Read the model definition and answer for the solid it produces. Units are mm, in the model's axes. A direction names the side the tool comes from. Coordinates: 2 decimals unless noted, no trailing zeros. Loops run counter-clockwise (first coordinate to the right, second up) from the corner with the lowest first, then second, coordinate; pieces in that order, holes last. Notation, with made-up numbers: (29.5, 37.5) -> (68.5, 37.5) arc R21 ccw to (68.5, 44.5) -> close; hole circle Ø5 at (-28, 44.25). An arc over 180 degrees is marked (long way). Answer in a Markdown table with one row per item.
```python
from build123d import *

# Parameters (mm, degrees)
ESQUISSE1_W              = 330
ESQUISSE1_H              = 370
CORP_DEPTH               = 40
CONG_AVANT_RADIUS        = 165
CONG_AVANT_LENGTH        = 40
TROU_POUR_ROUE_DEPTH     = 38
ESQUISSE4_R              = 2
TROU_POUR_ROULETTE_DEPTH = 50
TROU_POUR_BALAYEUR_DEPTH = 25
MOTEUR_PALE_DEPTH        = 6.3
ESQUISSE7_R              = 3
ENL_V_MAT_EXTRU_10_DEPTH = 6.3
ESQUISSE8_W              = 6
ESQUISSE8_H              = 3.075554286
ENL_V_MAT_EXTRU_11_DEPTH = 6.3
ESQUISSE9_R              = 19.061984771
ENL_V_MAT_EXTRU_12_DEPTH = 33


with BuildPart() as part:
    # Esquisse1 → corp (new body)
    with BuildSketch(Plane(origin=(0, 0, 0), x_dir=(1, 0, 0), z_dir=(0, 1, 0))):
        with Locations((165, 185)):
            Rectangle(ESQUISSE1_W, ESQUISSE1_H)
    extrude(amount=CORP_DEPTH)

    # congé avant: full round fillet: the end face becomes a half cylinder, R = half its width
    cong_avant_face = Plane((165, 20, -370), x_dir=(0, 1, 0), z_dir=(0, 0, -1))  # on the end face: x along it, z out of the body
    cong_avant_slab = cong_avant_face.offset(-CONG_AVANT_RADIUS / 2) * Box(CONG_AVANT_LENGTH, 2 * CONG_AVANT_RADIUS, CONG_AVANT_RADIUS, mode=Mode.PRIVATE)  # the body's end, R deep
    cong_avant_round = Plane((165, 20, -205), x_dir=(0, 0, -1), z_dir=(0, 1, 0)) * Cylinder(CONG_AVANT_RADIUS, CONG_AVANT_LENGTH, mode=Mode.PRIVATE)  # its axis R under the face
    add(cong_avant_slab - cong_avant_round, mode=Mode.SUBTRACT)

    # Esquisse3 → trou pour roue (cut)
    with BuildSketch(Plane(origin=(0, 40, 0), x_dir=(1, 0, 0), z_dir=(0, 1, 0))):
        Polygon((46, 124), (46, 135), (0, 135), (0, 0), (46, 0), (46, 59.234399469), (54.724206143, 59.234399469), (54.724206143, 75), (46, 75), (46, 95), (61, 95), (61, 124), align=None)
        Polygon((284, 95), (284, 75), (275.275793857, 75), (275.275793857, 59.234399469), (284, 59.234399469), (284, 0), (330, 0), (330, 135), (284, 135), (284, 124), (269, 124), (269, 95), align=None)
    extrude(amount=-TROU_POUR_ROUE_DEPTH, mode=Mode.SUBTRACT)

    # Esquisse4 → trou pour roulette (cut)
    with BuildSketch(Plane(origin=(0, 40, 0), x_dir=(1, 0, 0), z_dir=(0, 1, 0))):
        with Locations(Location((176.95, 352.458632269, 0), (0, 0, 270))):
            Circle(ESQUISSE4_R)
        with Locations(Location((176.95, 323.158632269, 0), (0, 0, 90))):
            Circle(ESQUISSE4_R)
        with Locations(Location((153.05, 323.158632269, 0), (0, 0, 270))):
            Circle(ESQUISSE4_R)
        with Locations(Location((153.05, 352.458632269, 0), (0, 0, 90))):
            Circle(ESQUISSE4_R)
    extrude(amount=-TROU_POUR_ROULETTE_DEPTH, mode=Mode.SUBTRACT)

    # Esquisse5 → Trou pour balayeur (cut)
    with BuildSketch(Plane(origin=(0, 40, 0), x_dir=(1, 0, 0), z_dir=(0, 1, 0))):
        with BuildLine():
            Line((90, 286), (240, 286))
            ThreePointArc((240, 286), (309.290964938, 239.701257427), (293.033008589, 157.966991411))
            Line((293.033008589, 157.966991411), (240, 104.933982822))
            Line((240, 104.933982822), (240, 0))
            Line((240, 0), (90, 0))
            Line((90, 0), (90, 104.933982822))
            Line((90, 104.933982822), (36.966991411, 157.966991411))
            ThreePointArc((36.966991411, 157.966991411), (20.709035062, 239.701257427), (90, 286))
        make_face()
    extrude(amount=-TROU_POUR_BALAYEUR_DEPTH, mode=Mode.SUBTRACT)

    # Esquisse6 → moteur pale (cut)
    with BuildSketch(Plane(origin=(0, 15, 0), x_dir=(1, 0, 0), z_dir=(0, 1, 0))):
        with BuildLine():
            Line((257.506073255, 187.1), (255.885842754, 211))
            ThreePointArc((255.885842754, 211), (251.445088501, 222.191160152), (240.245274455, 226.610043405))
            ThreePointArc((240.245274455, 226.610043405), (240.122739998, 226.602511903), (240, 226.6))
            ThreePointArc((240, 226.6), (229.088615697, 221.822854824), (224.114157246, 211))
            Line((224.114157246, 211), (222.506073255, 187.1))
            ThreePointArc((222.506073255, 187.1), (227.152012558, 174.508282489), (239.63580106, 169.57967959))
            ThreePointArc((239.63580106, 169.57967959), (239.977179555, 169.600029468), (240.318655983, 169.581395004))
            ThreePointArc((240.318655983, 169.581395004), (252.842661862, 174.484702191), (257.506073255, 187.1))
        make_face()
        with BuildLine():
            ThreePointArc((89.754725545, 226.610043405), (78.554911499, 222.191160152), (74.114157246, 211))
            Line((74.114157246, 211), (72.493926745, 187.1))
            ThreePointArc((72.493926745, 187.1), (77.157338138, 174.484702191), (89.681344017, 169.581395004))
            ThreePointArc((89.681344017, 169.581395004), (90.022820445, 169.600029468), (90.36419894, 169.57967959))
            ThreePointArc((90.36419894, 169.57967959), (102.847987442, 174.508282489), (107.493926745, 187.1))
            Line((107.493926745, 187.1), (105.885842754, 211))
            ThreePointArc((105.885842754, 211), (100.911384303, 221.822854824), (90, 226.6))
            ThreePointArc((90, 226.6), (89.877260002, 226.602511903), (89.754725545, 226.610043405))
        make_face()
    extrude(amount=-MOTEUR_PALE_DEPTH, mode=Mode.SUBTRACT)

    # Esquisse7 → Enlèv. mat.-Extru.10 (cut)
    with BuildSketch(Plane(origin=(0, 15, 0), x_dir=(1, 0, 0), z_dir=(0, 1, 0))):
        with Locations((240, 229.6)):
            Circle(ESQUISSE7_R)
        with Locations((90, 229.6)):
            Circle(ESQUISSE7_R)
        with Locations((90.015284108, 166.600038934)):
            Circle(ESQUISSE7_R)
        with Locations((239.984715892, 166.600038934)):
            Circle(ESQUISSE7_R)
    extrude(amount=-ENL_V_MAT_EXTRU_10_DEPTH, mode=Mode.SUBTRACT)

    # Esquisse8 → Enlèv. mat.-Extru.11 (cut)
    with BuildSketch(Plane(origin=(0, 15, 0), x_dir=(1, 0, 0), z_dir=(0, 1, 0))):
        Polygon((93, 229.6), (93, 226.178416603), (87, 226.178416603), (87, 226.449068216), (87, 229.6), align=None)
        Polygon((237, 226.178416603), (243, 226.178416603), (243, 226.449068216), (243, 229.6), (237, 229.6), align=None)
        with Locations((90.015284108, 168.137816077)):
            Rectangle(ESQUISSE8_W, ESQUISSE8_H)
        with Locations((239.984715892, 168.137816077)):
            Rectangle(ESQUISSE8_W, ESQUISSE8_H)
    extrude(amount=-ENL_V_MAT_EXTRU_11_DEPTH, mode=Mode.SUBTRACT)

    # Esquisse9 → Enlèv. mat.-Extru.12 (cut)
    with BuildSketch(Plane(origin=(0, 15, 0), x_dir=(1, 0, 0), z_dir=(0, 1, 0))):
        with Locations(Location((240.309161112, 188.734839537, 0), (0, 0, 307.62761802))):
            Circle(ESQUISSE9_R)
        with Locations(Location((89.690838888, 188.734839537, 0), (0, 0, 232.37238198))):
            Circle(ESQUISSE9_R)
    extrude(amount=-ENL_V_MAT_EXTRU_12_DEPTH, mode=Mode.SUBTRACT)


solid = part.part
```
1. A cutting plane is placed at A-A on z = -190.5. Give the vertices of the cut face in (x, y).
A:
| item | result |
|---|---|
| outline | (0, 0) -> (70.71, 0) -> (70.71, 15) -> (17.86, 15) -> (17.86, 40) -> (0, 40) -> close; (108.67, 0) -> (221.33, 0) -> (221.33, 15) -> (108.67, 15) -> close; (259.29, 0) -> (330, 0) -> (330, 40) -> (312.14, 40) -> (312.14, 15) -> (259.29, 15) -> close |
2. A cutting plane is placed at D-D on x = 210. Give the vertices of the cut face in (y, z).
A:
| item | result |
|---|---|
| outline | (0, -363.75) -> (40, -363.75) -> (40, -286) -> (15, -286) -> (15, 0) -> (0, 0) -> close |
3. A tool of negligible diameter and unlimited length cuts with its end or side. For faces 4 (the flat face through (307, 21, -135)), 5 (the cylindrical face through (308.81, 27.68, -240.84)), 6 (the flat face through (54, 21, -124)), from which of +Z, -Z, +X, -X, +Y, -Y can it reach the whole face along a straight path? Write none if from no direction.
A:
| item | result |
|---|---|
| face 4 | +Z, +X, +Y |
| face 5 | +Y |
| face 6 | -X, +Y |
4. Find the intervals of material crossed by probe 1 along X at (y, z) = (23, -63); probe 2 along X at (y, z) = (19, -94.5); probe 3 along Z at (x, y) = (51, 38.5), in increasing order.
A:
| item | result |
|---|---|
| probe 1 | x = 54.72 to 90, 240 to 275.28 |
| probe 2 | x = 46 to 90, 240 to 284 |
| probe 3 | z = -324.29 to -275.06, -143.93 to -124, -95 to -75, -59.23 to 0 |
5. A cutting plane is placed at C-C on z = -313.5. Give the vertices of the cut face in (x, y).
A:
| item | result |
|---|---|
| outline | (40.69, 0) -> (289.31, 0) -> (289.31, 40) -> (40.69, 40) -> close |
6. The mould has two halves that part along X. Classify faces 1 (the flat face through (266.888, 27.675, -131.822)), 2 (the flat face through (53, 21, -95)), 3 (the flat face through (61, 21, -109)): pulls with the +X half, pulls with the -X half, needs draft (parallel to the pull), parting line crosses it, or undercut.
A:
| item | result |
|---|---|
| face 1 | undercut |
| face 2 | needs draft |
| face 3 | pulls with the -X half |
7. Given pin 1 Ø2.5 at (y, z) = (11.5, -228.5) entering from +X; pin 2 Ø4.5 at (x, y) = (50, 20) entering from -Z; pin 3 Ø8 at (x, y) = (242, 14) entering from +Z; pin 4 Ø1.5 at (y, z) = (33.5, -70.5) entering from +X, each flat-ended and moving along its own axis, determine where each tip first touches the part or whether it passes through.
A:
| item | result |
|---|---|
| pin 1 | stops at x = 328.49 |
| pin 2 | stops at z = -325.47 |
| pin 3 | stops at z = 0 |
| pin 4 | stops at x = 275.28 |
8. A cutting plane is placed at B-B on x = 165. Give the vertices of the cut face in (y, z), and give its area (3 significant figures).
A:
| item | result |
|---|---|
| outline | (0, -370) -> (40, -370) -> (40, -286) -> (15, -286) -> (15, 0) -> (0, 0) -> close |
| area | 7,650 mm2 |
